Verification items for the finished model (mm, model axes). A direction names the side the tool comes from. Give positions to 0.01 mm unless a question says otherwise; leave off trailing zeros. Loops run counter-clockwise (first coordinate to the right, second up) from the corner with the lowest first, then second, coordinate; pieces in that order, holes last. Notation, with made-up numbers: M 71,64.25 L 106,64.25 A15 cw 106,88.25 Z; hole C 8,59.5 d9. An arc over 180 degrees is marked long. Answer in a Markdown table with one row per item.
```python
from build123d import *

# Parameters (mm, degrees)
F1_DEPTH = 25
F3_D     = 4.2
F3_DEPTH = 15
F3_TIP   = 1.2618073
F5_DEPTH = 25
F6_D     = 3
F6_DEPTH = 15
F6_TIP   = 0.9012909285


with BuildPart() as f1:
    # F0 (on Front) → F1 (new body)
    with BuildSketch(Plane.XZ):
        Polygon((0, 60), (0, 0), (35, 0), (35, 10), (8, 10), (8, 60), align=None)
    extrude(amount=F1_DEPTH)

    # F3
    with Locations(Plane.XY.offset(60)):
        with Locations((4, -5), (4, -20)):
            Hole(F3_D / 2, depth=F3_DEPTH)
            with Locations((0, 0, -(F3_DEPTH + F3_TIP / 2))):  # 118° drill point
                Cone(0, F3_D / 2, F3_TIP, mode=Mode.SUBTRACT)

    # F4 (on face) → F5 (cut)
    with BuildSketch(Plane.XY.offset(10)):
        with BuildLine():
            ThreePointArc((27, -15.8), (29.3334523779, -14.8334523779), (30.3, -12.5))
            ThreePointArc((30.3, -12.5), (29.3334523779, -10.1665476221), (27, -9.2))
            Line((27, -9.2), (27, -15.8))
        make_face()
        with BuildLine():
            Line((27, -15.8), (27, -9.2))
            ThreePointArc((27, -9.2), (23.7, -12.5), (27, -15.8))
        make_face()
        with BuildLine():
            ThreePointArc((27, -15.8), (23.7, -12.5), (27, -9.2))
            Line((27, -9.2), (17, -9.2))
            ThreePointArc((17, -9.2), (19.3334523779, -10.1665476221), (20.3, -12.5))
            ThreePointArc((20.3, -12.5), (19.3334523779, -14.8334523779), (17, -15.8))
            Line((17, -15.8), (27, -15.8))
        make_face()
        with BuildLine():
            ThreePointArc((20.3, -12.5), (19.3334523779, -10.1665476221), (17, -9.2))
            ThreePointArc((17, -9.2), (13.7, -12.5), (17, -15.8))
            ThreePointArc((17, -15.8), (19.3334523779, -14.8334523779), (20.3, -12.5))
        make_face()
    extrude(amount=-F5_DEPTH, mode=Mode.SUBTRACT)

    # F6
    with Locations(Plane.XY.offset(10)):
        with Locations((31, -21)):
            Hole(F6_D / 2, depth=F6_DEPTH)
            with Locations((0, 0, -(F6_DEPTH + F6_TIP / 2))):  # 118° drill point
                Cone(0, F6_D / 2, F6_TIP, mode=Mode.SUBTRACT)


solid = f1.part
```
Item 1: Scan lines: L1, parallel to Y at x = 4, z = 51.25; L2, parallel to X at y = -5, z = 56.75; L3, parallel to Z at x = 16, y = -21.25. Record each from-to range of solid material in increasing order. Write a range as [from, to].
Reported:
| item | result |
|---|---|
| L1 | y = [-25, -22.1], [-17.9, -7.1], [-2.9, 0] |
| L2 | x = [0, 1.9], [6.1, 8] |
| L3 | z = [0, 10] |
Item 2: Sectioned sample at C-C (x = 24). Record the cut outline in (y, z), and give its area (3 significant figures).
Reported:
| item | result |
|---|---|
| outline | M -25,0 L -15.8,0 L -15.8,10 L -25,10 Z; M -9.2,0 L 0,0 L 0,10 L -9.2,10 Z |
| area | 184 mm^2 |
Item 3: Tool access check on faces 5 (the cylindrical face through (4.273, -17.918, 52.395)), 6 (the flat face through (13, -12, 0)), 7 (the flat face through (7, 0, 23)), 8 (the flat face through (22, -9.2, 5)), 9 (the flat face through (8, -12, 35)). Record the directions out of +Z, -Z, +X, -X, +Y, -Y that give a thin tool (end or side, any length) a straight path to the whole face; none if there is none.
Reported:
| item | result |
|---|---|
| face 5 | +Z |
| face 6 | -Z, +X, -X, +Y, -Y |
| face 7 | +Z, -Z, +X, -X, +Y |
| face 8 | +Z, -Z |
| face 9 | +Z, +X, +Y, -Y |
Item 4: Sectioned sample at A-A (x = 31). Record the cut outline in (y, z), and give its area (3 significant figures).
Reported:
| item | result |
|---|---|
| outline | M -25,0 L -22.5,0 L -22.5,10 L -25,10 Z; M -19.5,0 L 0,0 L 0,10 L -19.5,10 Z |
| area | 220 mm^2 |
Item 5: Sectioned sample at D-D (z = 53.5). Record the cut outline in (x, y), and give its area (3 significant figures).
Reported:
| item | result |
|---|---|
| outline | M 0,-25 L 8,-25 L 8,0 L 0,0 Z; hole C 4,-20 d4.2; hole C 4,-5 d4.2 |
| area | 172 mm^2 |
Item 6: Release check for a two-part mould opening along X. For faces 1 (the flat face through (35, -12, 5)), 2 (the conical face through (4.2, -19.69, 43.96)), 3 (the flat face through (0, -12, 30)), 4 (the flat face through (22, -7, 10)) record: released by +X, released by -X, zero draft, split by the parting line, or undercut.
Reported:
| item | result |
|---|---|
| face 1 | released by +X |
| face 2 | undercut |
| face 3 | released by -X |
| face 4 | zero draft |
Item 7: Go/stop test with flat-tipped pins: pin 1 (6 mm diameter, centred on x = 12, y = -11.5, fed in from +Z); pin 2 (4 mm diameter, centred on x = 4, y = -20, fed in from +Z); pin 3 (2.5 mm diameter, centred on x = 4, y = -5, fed in from +Z). Record where each tip stops, or that it passes through.
Reported:
| item | result |
|---|---|
| pin 1 | stops at z = 10 |
| pin 2 | stops at z = 44.94 |
| pin 3 | stops at z = 44.49 |
Item 8: Sectioned sample at B-B (z = 5). Record the cut outline in (x, y), and give its area (3 significant figures).
Reported:
| item | result |
|---|---|
| outline | M 0,-25 L 35,-25 L 35,0 L 0,0 Z; hole M 17,-15.8 L 27,-15.8 A3.3 ccw 27,-9.2 L 17,-9.2 A3.3 ccw Z; hole C 31,-21 d3 |
| area | 768 mm^2 |
